```python
from build123d import *

# Parameters (mm, degrees)
SKETCH1_W           = 54.7
SKETCH1_H           = 54.7
BOSS_EXTRUDE1_DEPTH = 12.7
SKETCH2_W           = 15
SKETCH2_H           = 6.35
CUT_EXTRUDE1_DEPTH  = 41.710379512
SKETCH3_R           = 11
CUT_EXTRUDE2_DEPTH  = 41.710379512
CIRPATTERN1_COUNT   = 4


with BuildPart() as part:
    # Sketch1 → Boss-Extrude1 (new body)
    with BuildSketch(Plane.XY):
        Rectangle(SKETCH1_W, SKETCH1_H)
    extrude(amount=BOSS_EXTRUDE1_DEPTH)

    # Sketch2 → Cut-Extrude1 (cut, through all)
    with BuildSketch(Plane.XY.offset(12.7)):
        with Locations((0, 24.175)):
            Rectangle(SKETCH2_W, SKETCH2_H)
    cut_extrude1 = extrude(amount=-CUT_EXTRUDE1_DEPTH, mode=Mode.SUBTRACT)

    # Sketch3 → Cut-Extrude2 (cut, through all)
    with BuildSketch(Plane.XY.offset(12.7)):
        Circle(SKETCH3_R)
    extrude(amount=-CUT_EXTRUDE2_DEPTH, mode=Mode.SUBTRACT)

    # CirPattern1: Cut-Extrude1 ×4 about axis
    cirpattern1_axis = Axis((0, 0, 0), (0, 0, 1))
    for i in range(1, CIRPATTERN1_COUNT):
        add(cut_extrude1.rotate(cirpattern1_axis, i * 360 / CIRPATTERN1_COUNT), mode=Mode.SUBTRACT)


solid = part.part
```
Read the model definition and answer for the solid it produces. Units are mm, in the model's axes. A direction names the side the tool comes from. Give positions to 0.01 mm unless a question says otherwise; leave off trailing zeros. Write each loop counter-clockwise with the first axis right and the second up, starting at its lowest first coordinate (ties: lowest second). Pieces come first, ordered by that corner, then holes. Notation, with made-up numbers: (28.25, 34) -> (71.25, 34) arc R35 cw to (71.25, 69) -> close; hole circle Ø5 at (15.5, -29.75). An arc over 180 degrees is marked (long way). Answer as a JSON object with one key per item and string values.
1) For a pull along Y with two mould halves and no side action, classify faces 1 (the flat face through (-13, 0, 0)), 2 (the flat face through (24, 7.5, 6)), 3 (the flat face through (0, 21, 6)) as pulls with the +Y half, pulls with the -Y half, needs draft (parallel to the pull), parting line crosses it, or undercut.
Findings below:
{"face 1": "needs draft", "face 2": "undercut", "face 3": "pulls with the +Y half"}
2) Flat-ended cylindrical pins translate along their axes: pin 1 Ø6.5 at (x, z) = (0, 4.5) entering from -Y; pin 2 Ø6 at (x, z) = (-1, 6.5) entering from +Y; pin 3 Ø4 at (y, z) = (-3, 6) entering from +X. Find the tip coordinate at first contact, or state that the pin passes through.
Findings below:
{"pin 1": "stops at y = -21", "pin 2": "stops at y = 21", "pin 3": "stops at x = 21"}
3) A tool of negligible diameter and unlimited length cuts with its end or side. For faces 4 (the flat face through (7.5, -24, 6)), 5 (the flat face through (21, 0, 6)), 6 (the flat face through (-24, 7.5, 6)), from which of +Z, -Z, +X, -X, +Y, -Y can it reach the whole face along a straight path? Write none if from no direction.
Findings below:
{"face 4": "+Z, -Z, -Y", "face 5": "+Z, -Z, +X", "face 6": "+Z, -Z, -X"}
4) Section C-C on z = 10.25 is taken. Write down the section's boundary in (x, y).
Findings below:
{"outline": "(-27.35, -27.35) -> (-7.5, -27.35) -> (-7.5, -21) -> (7.5, -21) -> (7.5, -27.35) -> (27.35, -27.35) -> (27.35, -7.5) -> (21, -7.5) -> (21, 7.5) -> (27.35, 7.5) -> (27.35, 27.35) -> (7.5, 27.35) -> (7.5, 21) -> (-7.5, 21) -> (-7.5, 27.35) -> (-27.35, 27.35) -> (-27.35, 7.5) -> (-21, 7.5) -> (-21, -7.5) -> (-27.35, -7.5) -> close; hole circle Ø22 at (0, 0)"}
5) Section A-A on x = 0 is taken. Write down the section's boundary in (y, z).
Findings below:
{"outline": "(-21, 0) -> (-11, 0) -> (-11, 12.7) -> (-21, 12.7) -> close; (11, 0) -> (21, 0) -> (21, 12.7) -> (11, 12.7) -> close"}
6) Straight lines are drawn through the part: probe 1 along Y at (x, z) = (0, 10); probe 2 along X at (y, z) = (-23, 2.75); probe 3 along X at (y, z) = (0.5, 4.75). For each, find the intervals that lie inside material, in ascending order. Write a range as from..to.
Findings below:
{"probe 1": "y = -21..-11, 11..21", "probe 2": "x = -27.35..-7.5, 7.5..27.35", "probe 3": "x = -21..-10.99, 10.99..21"}
